from build123d import *

# Parameters (mm, degrees)
F5_DEPTH = 2.032


with BuildPart() as f1:
    # F0 (on Top) → F1 (revolve)
    with BuildSketch(Plane.XY):
        with BuildLine():
            Line((0, -12.7), (0, 12.7))
            ThreePointArc((0, 12.7), (-12.7, 0), (0, -12.7))
        make_face()
    revolve(axis=Axis((0, 0, 0), (0, -1, 0)))

    # F2 (on Top) + F3 (on Top) → F5 (join)
    with BuildSketch(Plane.XY):
        with BuildLine():
            add(Edge.make_bspline(
                [(-10.9918132212, 0), (-10.0577564866, 1.3559956811), (-22.0621618719, 5.2888968354), (-30.4974431762, -1.9048035346), (-12.0568089239, -1.5460833588), (-10.9918132212, 0)],
                knots=[0, 0, 0, 0, 0.3572272399, 0.5926955383, 1, 1, 1, 1], degree=3))
        make_face()
        with BuildLine():
            add(Edge.make_bspline(
                [(10.9918123134, 0), (11.1497141508, 2.1587421255), (30.4649991747, 20.3358374576), (23.1843343474, -3.6668601029), (17.44716018, 1.3878448006), (10.9036311724, -1.2055612974), (10.9918123134, 0)],
                knots=[0, 0, 0, 0, 0.3405356795, 0.6125251618, 0.8098259951, 1, 1, 1, 1], degree=3))
        make_face()
    with BuildSketch(Plane.XY):
        with BuildLine():
            add(Edge.make_bspline(
                [(-9.1440007091, -6.8580000661), (-10.6053034716, -6.3851140961), (-18.5643973908, -16.2954503659), (-10.7609585266, -17.8279019397), (-7.7549880842, -7.3074925323), (-9.1440007091, -6.8580000661)],
                knots=[0, 0, 0, 0, 0.3975006473, 0.622163571, 1, 1, 1, 1], degree=3))
        make_face()
        with BuildLine():
            add(Edge.make_bspline(
                [(9.1439997777, -8.0771995708), (8.2723022419, -8.9109545473), (12.9817126127, -15.8760986243), (17.8276538542, -11.670651754), (10.0357321804, -7.2242817894), (9.1439997777, -8.0771995708)],
                knots=[0, 0, 0, 0, 0.3776435433, 0.6136767969, 1, 1, 1, 1], degree=3))
        make_face()
    extrude(amount=F5_DEPTH)


solid = f1.part
CAD build for the part. Positions are in the model's coordinates, mm. A direction names the side the tool comes from. Coordinates: 2 decimals unless noted, no trailing zeros. Loops run counter-clockwise (first coordinate to the right, second up) from the corner with the lowest first, then second, coordinate; pieces in that order, holes last. Notation, with made-up numbers: (73.25, 9.5) -> (97.25, 9.5) arc R26 ccw to (97.25, 33.5) -> close; hole circle Ø6 at (35.25, 70). An arc over 180 degrees is marked (long way). One line per item, written item: value.
1. Slice it at A-A on z = 10. Write the cut outline in (x, y).
Answers:
outline: circle Ø15.66 at (0, 0)
2. Drill centre lines: line 1 (Z direction, x = 9.5, y = -9); line 2 (Z direction, x = -6.5, y = 10); line 3 (Y direction, x = -3.5, z = -5). Where is each one in solid material? Low to high. Write a range as [from, to].
Answers:
line 1: z = [0, 2.03]
line 2: z = [-4.36, 4.36]
line 3: y = [-11.14, 11.14]
3. Flat gauge pins, fed straight in: P1, Ø6, axis at x = 17, y = 4.5, coming from the -Z side; P2, Ø6, axis at x = 1, y = -1.5, coming from the -Z side; P3, Ø6, axis at x = 8, y = 9.5, coming from the -Z side. Where does each tip first touch, or does it go through?
Answers:
P1: stops at z = 0
P2: stops at z = -12.7
P3: stops at z = -8.52
4. Slice it at B-B on x = 8. Write the cut outline in (y, z).
Answers:
outline: circle Ø19.73 at (0, 0)
5. Which spindle directions (+Z, -Z, +X, -X, +Y, -Y) get a long thin tool onto all of the face, cutting with end or side? Do faces 1 (the face through (-12, -12, 2.032)), 2 (the face through (-12, -12, 0)), 3 (the face through (12, -11, 0)). Say none if no direction does.
Answers:
face 1: +Z, -X, -Y
face 2: -Z, -X, -Y
face 3: -Z, +X, -Y
